from build123d import *

# Parameters (mm, degrees)
F1_DEPTH     = 20
F2_T1_DEPTH  = 20
F2_T3_DEPTH  = 31.8767610709
F2_T5_DEPTH  = 38.9813299321
F2_T7_DEPTH  = 32.5
F2_T9_DEPTH  = 33.1624563251
F2_T11_DEPTH = 24.5256241898
F2_T13_DEPTH = 25.8546868248


# Not quite as in the source:
# - a fillet or chamfer that OpenCascade refuses, or shapes differently, is made with other operations: its cross-section is extruded or revolved along the edge and cut away or added


with BuildPart() as f1:
    # F0 (on Front) → F1 (new body)
    with BuildSketch(Plane.XZ):
        with BuildLine():
            Line((5, -39.686269666), (5, 0))
            Line((5, 0), (5, 49.7493718553))
            ThreePointArc((5, 49.7493718553), (-37.0809924355, -33.5410196625), (50, 0))
            Line((50, 0), (45, 0))
            Line((45, 0), (53.0514801827, 18.7251443562))
            Line((53.0514801827, 18.7251443562), (36.0514801827, 18.7251443562))
            Line((36.0514801827, 18.7251443562), (36.0514801827, 13.7251443562))
            Line((36.0514801827, 13.7251443562), (46.0514801827, 13.7251443562))
            Line((46.0514801827, 13.7251443562), (40, 0))
            Line((40, 0), (30, 0))
            Line((30, 0), (30, 18.7251443562))
            Line((30, 18.7251443562), (25, 18.7251443562))
            Line((25, 18.7251443562), (22, 16.2251443562))
            Line((22, 16.2251443562), (22, 13.7251443562))
            Line((22, 13.7251443562), (25, 13.7251443562))
            Line((25, 13.7251443562), (25, 0))
            Line((25, 0), (25, -10))
            Line((25, -10), (38.7298334621, -10))
            ThreePointArc((38.7298334621, -10), (26.4271306677, -30.0267674696), (5, -39.686269666))
        make_face()
        with BuildLine():
            Line((-5, 39.686269666), (-5, 0))
            Line((-5, 0), (-5, -39.686269666))
            ThreePointArc((-5, -39.686269666), (-40, 0), (-5, 39.686269666))
        make_face(mode=Mode.SUBTRACT)
    extrude(amount=F1_DEPTH)

    # F2: fillet of radius 2.5 on 15 edges, made by hand

    # F2_s2 → F2_t1 (join)
    with BuildSketch(Plane.XZ):
        with BuildLine():
            ThreePointArc((30, 2.5), (30.732233047, 0.732233047), (32.5, 0))
            Line((32.5, 0), (30, 0))
            Line((30, 0), (30, 2.5))
        make_face()
        with BuildLine():
            ThreePointArc((35.3553390593, -10), (37.3965805116, -11.056624327), (37.7123616633, -13.3333333333))
            ThreePointArc((37.7123616633, -13.3333333333), (38.2574185835, -11.677753351), (38.7298334621, -10))
            Line((38.7298334621, -10), (35.3553390593, -10))
        make_face()
        with BuildLine():
            ThreePointArc((-5, 36.7423461417), (-5.9188611699, 38.6788378149), (-8, 39.1918358845))
            ThreePointArc((-8, 39.1918358845), (-6.5046995466, 39.4675674929), (-5, 39.686269666))
            Line((-5, 39.686269666), (-5, 36.7423461417))
        make_face()
        with BuildLine():
            ThreePointArc((-5, -36.7423461417), (-5.9188611699, -38.6788378149), (-8, -39.1918358845))
            ThreePointArc((-8, -39.1918358845), (-6.5046995466, -39.4675674929), (-5, -39.686269666))
            Line((-5, -39.686269666), (-5, -36.7423461417))
        make_face()
        with BuildLine():
            ThreePointArc((5, -36.7423461417), (5.9188611699, -38.6788378149), (8, -39.1918358845))
            ThreePointArc((8, -39.1918358845), (6.5046995466, -39.4675674929), (5, -39.686269666))
            Line((5, -39.686269666), (5, -36.7423461417))
        make_face()
    extrude(amount=F2_T1_DEPTH)

    # F2_s4 → F2_t3 (cut)
    with BuildSketch(Plane.XZ.offset(-5.9383805354)):
        with BuildLine():
            ThreePointArc((5, 47.4341649025), (4.3136906253, 49.1547829066), (2.6315789474, 49.9306998974))
            ThreePointArc((2.6315789474, 49.9306998974), (3.8168664205, 49.8541024463), (5, 49.7493718553))
            Line((5, 49.7493718553), (5, 47.4341649025))
        make_face()
    extrude(amount=F2_T3_DEPTH, mode=Mode.SUBTRACT)

    # F2_s6 → F2_t5 (cut)
    with BuildSketch(Plane.XZ.offset(-9.490664966)):
        with BuildLine():
            ThreePointArc((51.5519019376, 15.2376093346), (51.3431363158, 17.6001284372), (49.2552141963, 18.7251443562))
            Line((49.2552141963, 18.7251443562), (53.0514801827, 18.7251443562))
            Line((53.0514801827, 18.7251443562), (51.5519019376, 15.2376093346))
        make_face()
    extrude(amount=F2_T5_DEPTH, mode=Mode.SUBTRACT)

    # F2_s8 → F2_t7 (cut)
    with BuildSketch(Plane.XZ.offset(-6.25)):
        with BuildLine():
            ThreePointArc((30, 16.2251443562), (29.267766953, 17.9929113092), (27.5, 18.7251443562))
            Line((27.5, 18.7251443562), (30, 18.7251443562))
            Line((30, 18.7251443562), (30, 16.2251443562))
        make_face()
        with BuildLine():
            ThreePointArc((22, 16.2251443562), (22.732233047, 14.4573774032), (24.5, 13.7251443562))
            Line((24.5, 13.7251443562), (22, 13.7251443562))
            Line((22, 13.7251443562), (22, 16.2251443562))
        make_face()
        with BuildLine():
            ThreePointArc((25, -7.5), (25.732233047, -9.267766953), (27.5, -10))
            Line((27.5, -10), (25, -10))
            Line((25, -10), (25, -7.5))
        make_face()
        with BuildLine():
            ThreePointArc((38.5514801827, 18.7251443562), (36.7837132297, 17.9929113092), (36.0514801827, 16.2251443562))
            Line((36.0514801827, 16.2251443562), (36.0514801827, 18.7251443562))
            Line((36.0514801827, 18.7251443562), (38.5514801827, 18.7251443562))
        make_face()
        with BuildLine():
            ThreePointArc((36.0514801827, 16.2251443562), (36.7837132297, 14.4573774032), (38.5514801827, 13.7251443562))
            Line((38.5514801827, 13.7251443562), (36.0514801827, 13.7251443562))
            Line((36.0514801827, 13.7251443562), (36.0514801827, 16.2251443562))
        make_face()
    extrude(amount=F2_T7_DEPTH, mode=Mode.SUBTRACT)

    # F2_s10 → F2_t9 (cut)
    with BuildSketch(Plane.XZ.offset(-6.5812281626)):
        with BuildLine():
            ThreePointArc((49.9306998974, -2.6315789474), (49.2478555278, -0.779381996), (47.4341649025, 0))
            Line((47.4341649025, 0), (50, 0))
            ThreePointArc((50, 0), (49.9826719717, -1.3162456325), (49.9306998974, -2.6315789474))
        make_face()
    extrude(amount=F2_T9_DEPTH, mode=Mode.SUBTRACT)

    # F2_s12 → F2_t11 (cut)
    with BuildSketch(Plane.XZ.offset(-2.2628120949)):
        with BuildLine():
            ThreePointArc((25.905124838, 18.7251443562), (25.0540616786, 18.5758233004), (24.3046638388, 18.1456975552))
            Line((24.3046638388, 18.1456975552), (25, 18.7251443562))
            Line((25, 18.7251443562), (25.905124838, 18.7251443562))
        make_face()
    extrude(amount=F2_T11_DEPTH, mode=Mode.SUBTRACT)

    # F2_s14 → F2_t13 (cut)
    with BuildSketch(Plane.XZ.offset(-2.9273434124)):
        with BuildLine():
            ThreePointArc((22.8995390008, 16.9747601902), (22.2360264469, 16.1145954819), (22, 15.0542069912))
            Line((22, 15.0542069912), (22, 16.2251443562))
            Line((22, 16.2251443562), (22.8995390008, 16.9747601902))
        make_face()
    extrude(amount=F2_T13_DEPTH, mode=Mode.SUBTRACT)


solid = f1.part
Build history of the part. All positions in model axes, mm. A direction names the side the tool comes from. Give positions to 0.01 mm unless a question says otherwise; leave off trailing zeros. Order: outer loops, then holes, each group sorted by start corner. A loop starts at its lowest first (then second) coordinate and runs counter-clockwise, first axis right, second up. Notation, with made-up numbers: M 67,-38 L 82,-38 A13 cw 82,-31 Z; hole C -18.75,49.25 d8. An arc over 180 degrees is marked long. Put each result on its own line as item: value.
Item 1: Wall check: probe 1 along X at (y, z) = (-7.5, -20); probe 2 along X at (y, z) = (-4.75, -33.5); probe 3 along X at (y, z) = (-17.75, 11) (3 decimals). Give the ranges that are in metal, low to high.
Results are:
probe 1: -45.83 to -34.64, -5 to 5, 34.64 to 45.83
probe 2: -37.12 to -21.86, -5 to 5, 21.86 to 37.12
probe 3: -48.775 to -38.458, -5 to 5, 25 to 30, 44.85 to 49.73
Item 2: Drop flat-ended pins along their axis: pin 1 Ø1 at (y, z) = (-14.5, -18) entering from +X; pin 2 Ø2 at (x, y) = (35.5, -11) entering from +Z; pin 3 Ø6 at (y, z) = (-12, 8) entering from +X; pin 4 Ø6 at (x, z) = (-37, -4.5) entering from +Y. Give the stop position or say it passes through.
Results are:
pin 1: x = 46.84
pin 2: z = 17.65
pin 3: x = 49.73
pin 4: y = 0
Item 3: Which spindle directions (+Z, -Z, +X, -X, +Y, -Y) get a long thin tool onto all of the face, cutting with end or side? Do faces 5 (the face through (44, -10, 18.725)), 6 (the face through (25, -10, 3)), 7 (the face through (49.267, -9.86, -0.8)). Say none if no direction does.
Results are:
face 5: +Z, +X, +Y, -Y
face 6: +Y, -Y
face 7: +X, +Y, -Y
Item 4: Cut at B-B on z = 27.5. Write the cut outline in (x, y), then the cut area to 3 significant figures.
Results are:
outline: M -41.76,-20 L -29.05,-20 L -29.05,0 L -41.76,0 Z; M -5,-20 L 5,-20 L 5,0 L -5,0 Z
area: 454 mm2
Item 5: Cut at C-C on x = 16. Write the cut outline in (y, z), then the cut area to 3 significant figures.
Results are:
outline: M -20,-47.37 L 0,-47.37 L 0,-36.66 L -20,-36.66 Z
area: 214 mm2
Item 6: Pull direction X, two halves, no side cores. Call faces 1 (the face through (36, -10, 0)), 2 (the face through (-38.25, -9.86, -32.2)), 3 (the face through (51.362, -9.86, 17.571)), 4 (the face through (-3, -20, -3)): +X half, -X half, draft (parallel to the pull), parting line (faces both ways), or undercut.
Results are:
face 1: undercut
face 2: parting line
face 3: +X half
face 4: draft
